```python
from build123d import *

# Parameters (mm, degrees)
F1_DEPTH = 25
F2_R     = 2.5
F3_DEPTH = 6.001


# Not quite as in the source:
# - a feature names something its author has since deleted; it is built from what else it names


with BuildPart() as f1:
    # F0 (on Front) → F1 (new body)
    with BuildSketch(Plane.XZ):
        with BuildLine():
            ThreePointArc((13, 0), (0, -13), (-13, 0))
            Line((-13, 0), (-13, -11))
            Line((-13, -11), (-29, -11))
            Line((-29, -11), (-29, -17))
            Line((-29, -17), (29, -17))
            Line((29, -17), (29, -11))
            Line((29, -11), (13, -11))
            Line((13, -11), (13, 0))
        make_face()
        with BuildLine():
            Line((-13, 12), (-13, 0))
            ThreePointArc((-13, 0), (0, -13), (13, 0))
            Line((13, 0), (13, 12))
            Line((13, 12), (7.25, 12))
            Line((7.25, 12), (7.25, 0))
            ThreePointArc((7.25, 0), (0, -7.25), (-7.25, 0))
            Line((-7.25, 0), (-7.25, 12))
            Line((-7.25, 12), (-13, 12))
        make_face()
    extrude(amount=F1_DEPTH)

    # F2 (on face) → F3 (cut, through all)
    with BuildSketch(Plane.XY.offset(-11)):
        with Locations((20.9999978542, -12.5)):
            Circle(F2_R)
        with Locations((-20.9999978542, -12.5)):
            Circle(F2_R)
    extrude(amount=-F3_DEPTH, mode=Mode.SUBTRACT)


solid = f1.part
```
Could you check a few things on this model? Use its own coordinates, in mm. A direction names the side the tool comes from. Round coordinates to 2 decimals unless told otherwise and drop trailing zeros. Loops run counter-clockwise (first coordinate to the right, second up) from the corner with the lowest first, then second, coordinate; pieces in that order, holes last.
Q1. I want a section at D-D (y = -17.25). Write out the boundary of the cut face in (x, z), and give its area (3 significant figures).
Q2. I want a section at C-C (z = -6.5). Write out the boundary of the cut face in (x, y), and give its area (3 significant figures).
Q3. Thinking about a two-plate mould opening in Y: for faces 4 (the cylindrical face through (20.46, -14.94, -13.96)), 5 (the cylindrical face through (0.16, -12.32, -7.25)), 6 (the flat face through (0, -25, -9)), which applies, pulls with the +Y half, pulls with the -Y half, needs draft (parallel to the pull), parting line crosses it, or undercut?
Q4. On a 3-axis mill with a long thin cutter (end or side, diameter ignored), from which of +Z, -Z, +X, -X, +Y, -Y can I reach the whole of each face in a straight line? I mean faces 1 (the flat face through (-7.25, -12, 6)), 2 (the flat face through (21.1, -9.5, -11)), 3 (the flat face through (-13, -12, 1)). Say none if no direction works.
Q5. I want a section at B-B (y = -12.5). Write out the boundary of the cut face in (x, z).
Q6. For P1, Ø5, axis at y = -3.5, z = 0, coming from the -X side; P2, Ø5, axis at x = 18.5, y = -16.5, coming from the +Z side; P3, Ø1.5, axis at y = -16, z = 9, coming from the +X side; P4, Ø4, axis at x = 6, y = -16.5, coming from the +Z side, each with a flat end and sliding along its axis, tell me the tip position at first contact or that it passes through.
Q7. I want a section at A-A (x = 21). Write out the boundary of the cut face in (y, z).
Q8. Please list where these lines run through material, in increasing order: L1, parallel to X at y = -13.25, z = 10; L2, parallel to Z at x = -16.5, y = -10.75; L3, parallel to X at y = -9.25, z = -6.5.
Answer below:
1. outline: (-29, -17) - (29, -17) - (29, -11) - (13, -11) - (13, 12) - (7.25, 12) - (7.25, 0) arc R7.25 cw to (-7.25, 0) - (-7.25, 12) - (-13, 12) - (-13, -11) - (-29, -11) - close
1. area: 689 mm2
2. outline: (-13, -25) - (-3.21, -25) - (-3.21, 0) - (-13, 0) - close; (3.21, -25) - (13, -25) - (13, 0) - (3.21, 0) - close
2. area: 489 mm2
3. face 4: undercut
3. face 5: needs draft
3. face 6: pulls with the -Y half
4. face 1: +Z, +Y, -Y
4. face 2: +Z, +X, +Y, -Y
4. face 3: +Z, -X, +Y, -Y
5. outline: (-29, -17) - (-23.5, -17) - (-23.5, -11) - (-29, -11) - close; (-18.5, -17) - (18.5, -17) - (18.5, -11) - (13, -11) - (13, 12) - (7.25, 12) - (7.25, 0) arc R7.25 cw to (-7.25, 0) - (-7.25, 12) - (-13, 12) - (-13, -11) - (-18.5, -11) - close; (23.5, -17) - (29, -17) - (29, -11) - (23.5, -11) - close
6. P1: stops at x = -13
6. P2: stops at z = -11
6. P3: stops at x = 13
6. P4: stops at z = 12
7. outline: (-25, -17) - (-15, -17) - (-15, -11) - (-25, -11) - close; (-10, -17) - (0, -17) - (0, -11) - (-10, -11) - close
8. L1: x = -13 to -7.25, 7.25 to 13
8. L2: z = -17 to -11
8. L3: x = -13 to -3.21, 3.21 to 13
